Here's how the part is built. I have some questions about the finished solid (model axes, mm). Face numbers are marked on the shaded views. A direction names the side the tool comes from. Round coordinates to 2 decimals unless told otherwise and drop trailing zeros. Order: outer loops, then holes, each group sorted by start corner. A loop starts at its lowest first (then second) coordinate and runs counter-clockwise, first axis right, second up. Notation, with made-up numbers: (47, 16.5) - (52, 16.5) arc R25 cw to (52, 49.5) - close; hole circle Ø1 at (-8, 64.5). An arc over 180 degrees is marked (long way). Answer as a JSON object with one key per item and string values.
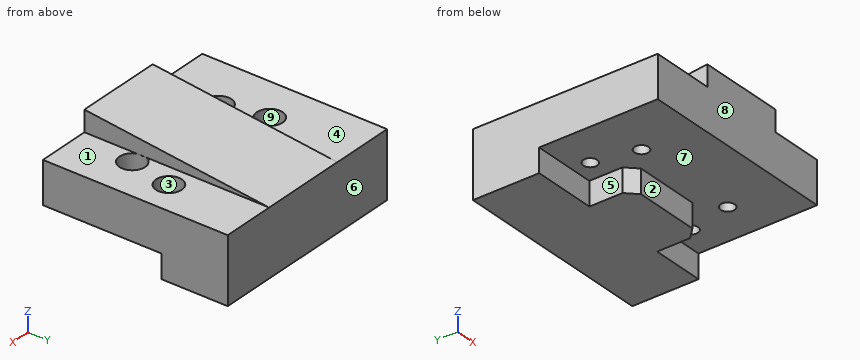
```python
from build123d import *

# Parameters (mm, degrees)
SKETCH1_R           = 1
BOSS_EXTRUDE2_DEPTH = 1.7
SKETCH2_R           = 1.85
BOSS_EXTRUDE3_DEPTH = 4.3
BOSS_EXTRUDE4_DEPTH = 3.4
BOSS_EXTRUDE5_DEPTH = 12.5


with BuildPart() as part:
    # Sketch1 → Boss-Extrude2 (new body)
    with BuildSketch(Plane.XY):
        Polygon((-16.230109425, 8.75), (-16.230109425, -1.75), (-16.230109425, -7), (-16.230109425, -17.75), (12.969890575, -17.75), (12.969890575, -7), (12.969890575, -1.75), (12.969890575, 8.75), align=None)
        with Locations((-10.080109425, -3.25)):
            Circle(SKETCH1_R, mode=Mode.SUBTRACT)
        with Locations((8.419890575, -3.25)):
            Circle(SKETCH1_R, mode=Mode.SUBTRACT)
        with Locations((-8.730109425, -9.55)):
            Circle(SKETCH1_R, mode=Mode.SUBTRACT)
        with Locations((7.069890575, -9.55)):
            Circle(SKETCH1_R, mode=Mode.SUBTRACT)
    extrude(amount=BOSS_EXTRUDE2_DEPTH)

    # Sketch2 → Boss-Extrude3 (add)
    with BuildSketch(Plane.XY.offset(1.7)):
        Polygon((-16.230109425, 8.75), (-16.230109425, -1.75), (-16.230109425, -7), (-16.230109425, -17.75), (12.969890575, -17.75), (12.969890575, -7), (12.969890575, -1.75), (12.969890575, 8.75), align=None)
        with Locations((-10.080109425, -3.25)):
            Circle(SKETCH2_R, mode=Mode.SUBTRACT)
        with Locations((8.419890575, -3.25)):
            Circle(SKETCH2_R, mode=Mode.SUBTRACT)
        with Locations((-8.730109425, -9.55)):
            Circle(SKETCH2_R, mode=Mode.SUBTRACT)
        with Locations((7.069890575, -9.55)):
            Circle(SKETCH2_R, mode=Mode.SUBTRACT)
    extrude(amount=BOSS_EXTRUDE3_DEPTH)

    # Sketch3 → Boss-Extrude4 (add)
    with BuildSketch(Plane(origin=(0, 0, 0), x_dir=(-1, 0, 0), z_dir=(0, 0, -1))):
        Polygon((-3.869890575, -7), (5.530109425, -7), (7.030109425, -5.5), (7.030109425, -0.75), (16.230109425, -0.75), (16.230109425, 8.75), (-12.969890575, 8.75), (-12.969890575, -0.75), (-5.369890575, -0.75), (-5.369890575, -5.5), align=None)
    extrude(amount=BOSS_EXTRUDE4_DEPTH)

    # Sketch4 → Boss-Extrude5 (add)
    with BuildSketch(Plane(origin=(5.369890575, 0, 0), x_dir=(0, 0, -1), z_dir=(1, 0, 0))):
        Polygon((-6, -17.75), (-6, 8.75), (-9, -17.75), align=None)
    extrude(amount=-BOSS_EXTRUDE5_DEPTH)


solid = part.part
```
1. Thinking about a two-plate mould opening in Y: for the marked faces 6, 7, 8 and 9, which applies, pulls with the +Y half, pulls with the -Y half, needs draft (parallel to the pull), parting line crosses it, or undercut?
Responses:
{"face 6": "pulls with the +Y half", "face 7": "needs draft", "face 8": "pulls with the -Y half", "face 9": "undercut"}
2. Imagine slicing it at C-C (x = 3.25). List the corners of the cut face in (y, z) for me, plus the area to 3 significant figures.
Responses:
{"outline": "(-17.75, 0) - (-7, 0) - (-7, -3.4) - (8.75, -3.4) - (8.75, 6) - (-17.75, 9) - close", "area": "252 mm2"}
3. For P1, Ø2.5, axis at x = -8.73, y = -9.55, coming from the -Z side; P2, Ø4, axis at x = -8.5, y = -9, coming from the +Z side; P3, Ø2.5, axis at x = 8, y = -0.5, coming from the +Z side; P4, Ø3.5, axis at y = -4, z = -1.5, coming from the +X side, each with a flat end and sliding along its axis, tell me the tip position at first contact or that it passes through.
Responses:
{"P1": "z = 0", "P2": "z = 8.17", "P3": "z = 6", "P4": "x = 12.97"}
4. Imagine slicing it at A-A (y = -3.25). List the corners of the cut face in (x, z) for me, plus the area to 3 significant figures.
Responses:
{"outline": "(-16.23, 0) - (-11.08, 0) - (-11.08, 1.7) - (-11.93, 1.7) - (-11.93, 6) - (-16.23, 6) - close; (-9.08, 0) - (-7.03, 0) - (-7.03, -3.4) - (5.37, -3.4) - (5.37, 0) - (7.42, 0) - (7.42, 1.7) - (6.57, 1.7) - (6.57, 6) - (5.37, 6) - (5.37, 7.36) - (-7.13, 7.36) - (-7.13, 6) - (-8.23, 6) - (-8.23, 1.7) - (-9.08, 1.7) - close; (9.42, 0) - (12.97, 0) - (12.97, 6) - (10.27, 6) - (10.27, 1.7) - (9.42, 1.7) - close", "area": "196 mm2"}
5. Imagine slicing it at B-B (z = 5). List the corners of the cut face in (x, y) for me.
Responses:
{"outline": "(-16.23, -17.75) - (12.97, -17.75) - (12.97, 8.75) - (-16.23, 8.75) - close; hole circle Ø3.7 at (-10.08, -3.25); hole circle Ø3.7 at (-8.73, -9.55); hole circle Ø3.7 at (7.07, -9.55); hole circle Ø3.7 at (8.42, -3.25)"}
6. For the marked faces 1, 2, 3, 4 and 5, which set-ups out of +Z, -Z, +X, -X, +Y, -Y let a thin tool reach every point of the face, with its end or its side?
Responses:
{"face 1": "+Z, +X, +Y, -Y", "face 2": "-Z, +X, -X, -Y", "face 3": "+Z", "face 4": "+Z, -X, +Y, -Y", "face 5": "-Z, -X, -Y"}
7. Imagine slicing it at D-D (y = -9.55). List the corners of the cut face in (x, z) for me.
Responses:
{"outline": "(-16.23, 0) - (-9.73, 0) - (-9.73, 1.7) - (-10.58, 1.7) - (-10.58, 6) - (-16.23, 6) - close; (-7.73, 0) - (6.07, 0) - (6.07, 1.7) - (5.22, 1.7) - (5.22, 6) - (5.37, 6) - (5.37, 8.07) - (-7.13, 8.07) - (-7.13, 6) - (-6.88, 6) - (-6.88, 1.7) - (-7.73, 1.7) - close; (8.07, 0) - (12.97, 0) - (12.97, 6) - (8.92, 6) - (8.92, 1.7) - (8.07, 1.7) - close"}
8. If I drill on L1, parallel to X at y = -4.5, z = 5; L2, parallel to X at y = -3.75, z = 3; L3, parallel to Y at x = -14, z = -0.25, over which ranges is the centre line in solid material (lowest first)? Write a range as [from, to].
Responses:
{"L1": "[-16.23, -11.44], [-8.72, 7.06], [9.78, 12.97]", "L2": "[-16.23, -11.86], [-8.3, 6.64], [10.2, 12.97]", "L3": "[-0.75, 8.75]"}
